Input: part model. Units: mm. Frame: model coordinates. A direction names the side the tool comes from. Coordinates: 2 decimals unless noted, no trailing zeros. Order: outer loops, then holes, each group sorted by start corner. A loop starts at its lowest first (then second) coordinate and runs counter-clockwise, first axis right, second up. Notation, with made-up numbers: (-16, 21) -> (15, 21) arc R23 ccw to (15, 53) -> close; hole circle Ø3 at (-29.5, 49.5). An arc over 180 degrees is marked (long way). One line per question, with ' | ' between items.
Autodesk Inventor part; units mm, degrees
ref_plane "YZ Plane" through (0, 0, 0) normal (1, 0, 0) x (0, 1, 0)
ref_plane "XZ Plane" through (0, 0, 0) normal (0, 1, 0) x (-1, 0, 0)
ref_plane "XY Plane" through (0, 0, 0) normal (0, 0, 1) x (1, 0, 0)
sketch "Sketch1" plane through (0, 0, 0) normal (1, 0, 0) x (0, 1, 0)
  line L0 (0, 0) -> (0, -104)
  line L1 (79.3684, 0) -> (0, -104)
  line L2 (79.3684, 0) -> (0, 0)
  line L3 (0, -104) -> (0, -104)
  line L4 (0, -104) -> (0, -106)
  line L5 (0, -106) -> (0, -106)
  line L6 (12, -88.2759) -> (12, -121.4374)
  line L7 (17, -106) -> (0, -106)
  line L8 (17, -104) -> (0, -104)
  line L9 (85.6581, 0) -> (17, -89.9658)
  line L10 (105.5294, 0) -> (79.3684, 0)
  line L11 (17, -89.9658) -> (17, -119.3457)
  circle A0 centre (12, -106) radius 2
  point P0 (12, -104)
  point P1 (14, -106)
  dimension "d5" = 79.3684
  dimension "d6" = 104
  dimension "d7" = 12
  dimension "d8" = 88.2759
  dimension "d9" = 0
  dimension "d11" = 2
  dimension "d12" = 5
  dimension "d13" = 5
extrude "Extrusion1" add sketch "Sketch1" along normal blind 2 contours L10 L9 L11 L8 L6 L1 | L8 L11 L7 A0
sketch "Sketch2" plane through (2, 0, 0) normal (1, 0, 0) x (0, 0, -1)
  line L0 (0, 85.6581) -> (0, 79.3684)
  line L1 (0, 80.6581) -> (89.9658, 12)
  line L2 (88.2759, 12) -> (104, 12)
  line L3 (0, 79.3684) -> (88.2759, 12)
  line L4 (102.4983, 12) -> (102.4983, 15.9748)
  line L5 (89.9658, 17) -> (0, 85.6581)
  line L6 (106, 14) -> (106, 17)
  line L7 (106, 15.9748) -> (91.3092, 15.9748)
  line L8 (0, 85.6581) -> (91.3092, 15.9748)
  line L9 (106, 15.9748) -> (106, 17)
  line L10 (106, 17) -> (89.9658, 17)
  line L11 (106, 15.9748) -> (106, 17)
  line L12 (106, 17) -> (89.9658, 17)
  point P0 (0, 0)
  dimension "d18" = 5
  dimension "d19" = 3.9748
  dimension "d20" = 3.9748
extrude "Extrusion2" cut sketch "Sketch2" against normal blind 2 contours L1 L2 L3 L0 | L10 L6 L7 L8
sketch "Sketch3" plane through (2, 0, 0) normal (1, 0, 0) x (0, 0, -1)
  line L0 (91.3092, 15.9748) -> (0, 85.6581)
  line L1 (0, 85.6581) -> (91.3092, 15.9748)
  line L2 (91.3092, 15.9748) -> (106, 15.9748)
  line L3 (91.3092, 15.9748) -> (106, 15.9748)
  arc A0 (106, 14) -> (104, 12) centre (106, 12) ccw
  line L4 (106, 15.9748) -> (106, 14)
  circle A1 centre (106, 12) radius 2
  line L5 (89.9658, 12) -> (104, 12)
  line L6 (89.9658, 12) -> (104, 12)
  line L7 (0, 85.6581) -> (0, 80.6581)
  line L8 (0, 85.6581) -> (0, 80.6581)
  line L9 (0, 80.6581) -> (89.9658, 12)
  line L10 (0, 83.1581) -> (-58.5, 83.1581)
  line L11 (0, 85.6581) -> (0, 80.6581)
  line L12 (-58.5, 83.1581) -> (-58.5, 115.0333)
  line L13 (106, 14) -> (104, 14)
  line L14 (104, 14) -> (104, -16)
  line L15 (104, -16) -> (106, -16)
  line L16 (106, -16) -> (106, 14)
  line L17 (89.9658, 12) -> (89.9658, 145)
  line L18 (0, 83.1581) -> (89.9658, 83.1581)
  point P0 (0, 0)
  dimension "d21" = 58.5
  dimension "d32" = 30
  dimension "d42" = 89.9658
revolve "Revolution1" add sketch "Sketch3" angle 90 about axis through (2, 83.1581, 58.5) along (0, -1, 0) contours L2 L4 L13 L14 L5 L17 L0 | L17 L9 L7 L18 L0 | L18 L7 L0 | L16 A1 A0 | A0 L14 L13 | A1 L16 L15 L14
sketch "Sketch14" plane through (166.5, -16, 58.5) normal (0, 0, 1) x (1, 0, 0)
  line L0 (-14.6908, 31.9748) -> (-106, 101.6581)
  line L1 (-106, 96.6581) -> (-16.0342, 28)
  line L2 (-106, 101.6581) -> (-106, 96.6581)
  line L3 (-16.0342, 28) -> (-2, 28)
  line L4 (-106, 96.6581) -> (-16.0342, 28)
  point P0 (-166.5, 16)
sketch "Sketch4" plane through (60.5, 80.6581, 58.5) normal (0, 0, 1) x (1, 0, 0)
  line L0 (0, 5) -> (0, 0)
  line L1 (0, 5) -> (0, 0)
  line L2 (0, 0) -> (89.9658, -68.6581)
  line L3 (0, 0) -> (89.9658, -68.6581)
  line L4 (89.9658, -68.6581) -> (104, -68.6581)
  line L5 (89.9658, -68.6581) -> (104, -68.6581)
  line L6 (106, -66.6581) -> (106, -64.6834)
  line L7 (106, -66.6581) -> (106, -64.6834)
  line L8 (91.3092, -64.6834) -> (0, 5)
  line L9 (106, -64.6834) -> (91.3092, -64.6834)
  line L10 (91.3092, -64.6834) -> (0, 5)
  arc A0 (106, -66.6581) -> (104, -68.6581) centre (106, -68.6581) ccw
  circle A1 centre (106, -68.6581) radius 2
  point P0 (-60.5, -80.6581)
extrude "Extrusion3" add sketch "Sketch4" along normal blind 2 contours L8 L9 L6 A0 L4 L2 L0
sketch "Sketch5" plane through (60.5, 80.6581, 60.5) normal (0, 0, 1) x (1, 0, 0)
  line L0 (0, 5) -> (0, 0)
  line L1 (0, 2.5) -> (90.621, -66.6581)
  line L2 (-58.5, -66.6581) -> (106, -66.6581)
  line L3 (91.3092, -64.6834) -> (0, 5)
  line L4 (90.621, -66.6581) -> (106, -66.6581)
  line L5 (106, -66.6581) -> (106, -64.6834)
  line L6 (106, -64.6834) -> (91.3092, -64.6834)
  line L7 (106, -64.6834) -> (91.3092, -64.6834)
  line L8 (-58.5, 5) -> (0, 5)
  line L9 (91.3092, -64.6834) -> (0, 5)
  line L10 (0, 5) -> (0, 2.5)
  line L11 (0, 0) -> (89.9658, -68.6581)
  line L12 (89.9658, -68.6581) -> (106, -68.6581)
  line L13 (89.9658, -68.6581) -> (104, -68.6581)
  line L14 (106, -68.6581) -> (106, -66.6581)
  line L15 (90.621, -66.6581) -> (0, 2.5)
  line L16 (0, 0) -> (89.9658, -68.6581)
  point P0 (-60.5, -80.6581)
extrude "Extrusion4" cut sketch "Sketch5" against normal blind 2 contours L1 L2 L11 L0 | L2 L14 L12 L11
sketch "Sketch6" plane through (0, 0, 0) normal (-1, 0, 0) x (0, 0, 1)
  line L0 (0, 85.6581) -> (0, 80.6581)
  line L1 (0, 83.1581) -> (-90.621, 14)
  line L2 (-106, 14) -> (58.5, 14)
  line L3 (-91.3092, 15.9748) -> (0, 85.6581)
  line L4 (-106, 14) -> (-106, 15.9748)
  line L5 (-90.621, 14) -> (-106, 14)
  line L6 (-106, 14) -> (-106, 15.9748)
  line L7 (-106, 15.9748) -> (-91.3092, 15.9748)
  line L8 (0, 85.6581) -> (0, 83.1581)
  line L9 (-89.9658, 12) -> (58.5, 12)
  line L10 (-89.9658, 12) -> (-106, 12)
  line L11 (-104, 12) -> (58.5, 12)
  line L12 (-106, 12) -> (-106, 14)
  line L13 (-90.621, 14) -> (0, 83.1581)
  line L14 (0, 80.6581) -> (-89.9658, 12)
  point P0 (0, 0)
extrude "Extrusion5" cut sketch "Sketch6" against normal blind 2 contours L0 L14 L2 L1 | L2 L14 L10 L12
equation "\"d19\" = d20"
properties part number "Cover_v1"
1. Cut plane A-A, the plane y = 0.5. Return loops of the section in (x, z), and give its area (3 significant figures).
Recorded:
outline: (2, -106) arc R164.5 ccw to (166.5, 58.5) -> (164.5, 58.5) arc R162.5 cw to (2, -104) -> close | area: 514 mm^2
2. Ray query, line 1 (Y direction, x = 117, z = -42); line 2 (Y direction, x = 135.5, z = 49); line 3 (Z direction, x = 67.5, y = 28). Return the intervals inside material, ascending. Write a range as [from, to].
Recorded:
line 1: y = [12, 15.97] | line 2: y = [23.16, 28.16] | line 3: z = [-58.46, -50.89]
3. Access query for faces 1 (the face through (108, 15.975, -49)), 2 (the face through (115.634, -2.196, -57.661)), 3 (the face through (117.033, -0.236, -59.091)). Directions: +Z, -Z, +X, -X, +Y, -Y. A direction counts if a zero-diameter tool reaches every point of the face in a straight line with its end or side. Return the directions, or none.
Recorded:
face 1: -Z, +X, +Y | face 2: +Z, -X, -Y | face 3: -Z, +X, +Y, -Y
4. Pin query (flat end, axial travel): pin 1 Ø1.6 at (x, z) = (155.5, 59.5) entering from +Y; pin 2 Ø10 at (y, z) = (30.5, 16.5) entering from -X; pin 3 Ø1.5 at (x, y) = (58, 2) entering from -Z. Return the tip coordinate at first contact, or that it passes through.
Recorded:
pin 1: stops at y = 15.97 | pin 2: stops at x = 111.66 | pin 3: stops at z = -96.44
